Autodesk Inventor part; units mm, degrees
ref_plane "YZ Plane" through (0, 0, 0) normal (1, 0, 0) x (0, 1, 0)
ref_plane "XZ Plane" through (0, 0, 0) normal (0, 1, 0) x (-1, 0, 0)
ref_plane "XY Plane" through (0, 0, 0) normal (0, 0, 1) x (1, 0, 0)
sketch "Sketch1" plane through (0, 0, 0) normal (0, 1, 0) x (-1, 0, 0)
  circle A0 centre (0, -48.85) radius 21
  line L0 (0, -48.85) -> (0, 0) construction
  circle A1 centre (42.3053, -24.425) radius 21
  circle A2 centre (42.3053, 24.425) radius 21
  circle A3 centre (0, 48.85) radius 21
  circle A4 centre (-42.3053, 24.425) radius 21
  circle A5 centre (-42.3053, -24.425) radius 21
  circle A6 centre (0, 0) radius 76.2
  circle A7 centre (0, 0) radius 5.08
  dimension "d0" = 42
  dimension "d2" = 48.85
  dimension "d5" = 360
  dimension "d7" = 152.4
  dimension "d8" = 10.16
extrude "Extrusion1" add sketch "Sketch1" along normal blind 6.35
sketch "Sketch2" plane through (0, 6.35, 0) normal (0, 1, 0) x (1, 0, 0)
  circle A0 centre (0, 0) radius 5.08
  line L0 (-8.89, 0) -> (8.89, 0) construction
  dimension "d11" = 17.78
hole "Hole1" at (-8.89, 6.35, 0) at (8.89, 6.35, 0) direction (0, -1, 0) diameter 4.3053 end through all
sketch "Sketch3" plane through (0, 6.35, 0) normal (0, 1, 0) x (1, 0, 0)
  circle A0 centre (-8.89, 0) radius 2.1526
  circle A1 centre (0, 0) radius 5.08
  circle A2 centre (0, 0) radius 76.2
  line L0 (-32.667, 57.5809) -> (-33.533, 57.0809)
  line L1 (-33.533, 57.0809) -> (-39.803, 67.9408)
  line L2 (-39.803, 67.9408) -> (-38.937, 68.4408)
  line L3 (-38.937, 68.4408) -> (-32.667, 57.5809)
  line L4 (-33.1, 57.3309) -> (-39.37, 68.1908) construction
  line L5 (0, 0) -> (-8.89, 0) construction
  dimension "d21" = 10
  dimension "d22" = 1
  dimension "d23" = 60
  dimension "d29" = 2.54
extrude "Extrusion2" cut sketch "Sketch3" against normal through all contours L3 L0 L1 A2 | A2 L1 L2 L3 picked at (-34.8148, 60.1898)
pattern_circular "Circular Pattern1" count 6 over 360 about axis through (0, -10, 0) along (0, 1, 0) of "Extrusion2"
properties part number "carousel"
Here's how the part is built. I have some questions about the finished solid (model axes, mm). A direction names the side the tool comes from. Round coordinates to 2 decimals unless told otherwise and drop trailing zeros. Order: outer loops, then holes, each group sorted by start corner. A loop starts at its lowest first (then second) coordinate and runs counter-clockwise, first axis right, second up. Notation, with made-up numbers: (57.25, -22) -> (87.25, -22) arc R19 cw to (87.25, 2) -> close; hole circle Ø2 at (-34.75, 48.25). An arc over 180 degrees is marked (long way). Return JSON: item names as keys, results as strings.
Q1. If we section it at B-B on z = -21: List the corners of the cut face in (x, y) for me.
Filled sheet:
{"outline": "(-73.25, 0) -> (-63.02, 0) -> (-63.02, 6.35) -> (-73.25, 6.35) -> close; (-21.59, 0) -> (21.59, 0) -> (21.59, 6.35) -> (-21.59, 6.35) -> close; (63.02, 0) -> (73.25, 0) -> (73.25, 6.35) -> (63.02, 6.35) -> close"}
Q2. If we section it at A-A on x = 17.5: List the corners of the cut face in (y, z) for me, plus the area to 3 significant figures.
Filled sheet:
{"outline": "(0, -74.16) -> (6.35, -74.16) -> (6.35, -60.46) -> (0, -60.46) -> close; (0, -37.24) -> (6.35, -37.24) -> (6.35, 37.24) -> (0, 37.24) -> close; (0, 60.46) -> (6.35, 60.46) -> (6.35, 74.16) -> (0, 74.16) -> close", "area": "647 mm^2"}
Q3. If we mould it in two halves opening along Z, with no side actions, what happens to faces 1 (the cylindrical face through (65.7, 3.1, -38.6)), 2 (the flat face through (-16, 6.35, 1)), 3 (the flat face through (35.2, 3.22, 61.97))? For each: released by +Z, released by -Z, zero draft, split by the parting line, or undercut.
Filled sheet:
{"face 1": "released by -Z", "face 2": "zero draft", "face 3": "undercut"}
Q4. I need wall thicknesses on line 1 along Z through (x, y) = (0, 1.75); line 2 along Z through (x, y) = (26, 4); line 3 along X through (y, z) = (4.5, -22). Which ranges of each line are inside material? Lowest first, please. Write a range as from..to.
Filled sheet:
{"line 1": "z = -76.2..-69.85, -27.85..-5.08, 5.08..27.85, 69.85..76.2", "line 2": "z = -71.63..-37.66, -11.19..11.19, 37.66..71.63", "line 3": "x = -72.96..-63.16, -21.45..21.45, 63.16..72.96"}
Q5. For pin 1 Ø1.9 at (x, y) = (-69, 2) entering from +Z; pin 2 Ø5.5 at (x, z) = (-8.89, 0) entering from -Y; pin 3 Ø0.8 at (y, z) = (2, 0) entering from +X; pin 4 Ø1.9 at (x, y) = (-70, 4) entering from -Z, each with a flat end and sliding along its axis, tell me the tip position at first contact or that it passes through.
Filled sheet:
{"pin 1": "stops at z = 34.29", "pin 2": "stops at y = 0", "pin 3": "stops at x = 66.2", "pin 4": "stops at z = -32.23"}
Q6. If we section it at C-C on y = 1.75: Give the number of separate pieces and of enclosed holes in the cut face, plus the area to 3 significant figures.
Filled sheet:
{"separate pieces": "1", "enclosed holes": "9", "area": "9,760 mm^2"}
Q7. If we section it at D-D on z = -48.85: List the corners of the cut face in (x, y) for me.
Filled sheet:
{"outline": "(-58.48, 0) -> (-21, 0) -> (-21, 6.35) -> (-58.48, 6.35) -> close; (21, 0) -> (58.48, 0) -> (58.48, 6.35) -> (21, 6.35) -> close"}
Q8. Which directions (+Z, -Z, +X, -X, +Y, -Y) give clear straight access to the entire face, cutting with the end or side of a thin tool? Please do faces 4 (the flat face through (35.13, 3.22, -61.85)), 5 (the cylindrical face through (-65.7, 3.1, 38.6)).
Filled sheet:
{"face 4": "+Y, -Y", "face 5": "+Z, -X, +Y, -Y"}
